Autodesk Inventor part; units mm, degrees
ref_plane "YZ Plane" through (0, 0, 0) normal (1, 0, 0) x (0, 1, 0)
ref_plane "XZ Plane" through (0, 0, 0) normal (0, 1, 0) x (-1, 0, 0)
ref_plane "XY Plane" through (0, 0, 0) normal (0, 0, 1) x (1, 0, 0)
sketch "Sketch1" plane through (0, 0, 0) normal (0, 1, 0) x (-1, 0, 0)
  circle A0 centre (0, 0) radius 6.35
  line L0 (22, 0) -> (6.76, 15.24)
  line L1 (6.76, 15.24) -> (-15.24, 9.525)
  line L2 (-15.24, 9.525) -> (-15.24, 0)
  line L3 (22, 0) -> (0, 0)
  line L4 (22, 0) -> (6.76, -15.24)
  line L5 (6.76, -15.24) -> (-15.24, -9.525)
  line L6 (-15.24, -9.525) -> (-15.24, 0)
  dimension "d0" = 12.7
  dimension "d1" = 22
  dimension "d2" = 15.24
  dimension "d3" = 45
  dimension "d4" = 15.24
  dimension "d5" = 9.525
extrude "Extrusion1" add sketch "Sketch1" along normal blind 6.35
fillet "Fillet1" radius 1.27 5 edges at (-22, 3.175, 0) (-6.76, 3.175, 15.24) (-6.76, 3.175, -15.24) (15.24, 3.175, 9.525) (15.24, 3.175, -9.525)
properties part number "ALIGNMENT JIG 2SCREEN"
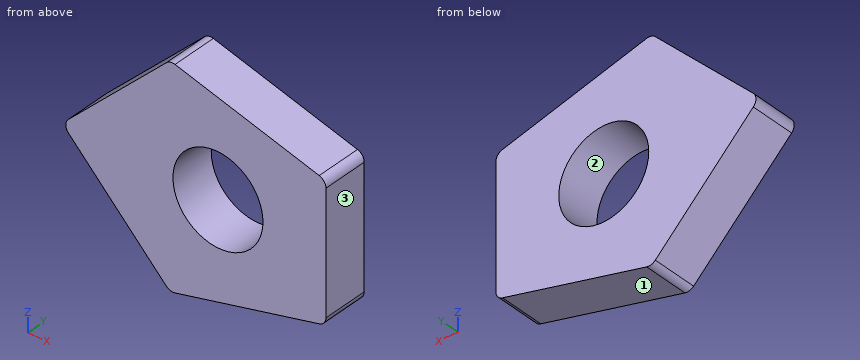
The listing builds one solid part. Answer for the finished solid, in the listing's coordinates (mm). Face numbers are marked on the shaded views. Coordinates: 2 decimals unless noted, no trailing zeros. Order: outer loops, then holes, each group sorted by start corner. A loop starts at its lowest first (then second) coordinate and runs counter-clockwise, first axis right, second up.
Q1. A cutting plane is placed at C-C, the plane x = -0.5. Write down the section's boundary in (y, z), and give its area (3 significant figures).
Q2. Consider line 1 (Z direction, x = -4.5, y = 1); line 2 (Z direction, x = 0, y = 2.25); line 3 (X direction, y = 2, z = -2.5). Determine where each line is inside the solid, lowest interval first.
Q3. A cutting plane is placed at A-A, the plane y = 1. Write down the section's boundary in (x, z), and give its area (3 significant figures).
Q4. Given P1, Ø1, axis at x = 1.5, y = 5, coming from the -Z side; P2, Ø3, axis at x = -8, y = 1, coming from the -Z side, each flat-ended and moving along its own axis, determine where each tip first touches the part or whether it passes through.
Q5. For a pull along Z with two mould halves and no side action, classify the marked faces 1, 2 and 3 as pulls with the +Z half, pulls with the -Z half, needs draft (parallel to the pull), parting line crosses it, or undercut.
Q6. A cutting plane is placed at D-D, the plane x = -11.5. Write down the section's boundary in (y, z), and give its area (3 significant figures).
Q7. A cutting plane is placed at B-B, the plane z = 0. Write down the section's boundary in (x, y).
Answers follow:
1. outline: (0, -13.61) - (6.35, -13.61) - (6.35, -6.33) - (0, -6.33) - close; (0, 6.33) - (6.35, 6.33) - (6.35, 13.61) - (0, 13.61) - close
1. area: 92.5 mm2
2. line 1: z = -14.65 to -4.48, 4.48 to 14.65
2. line 2: z = -13.48 to -6.35, 6.35 to 13.48
2. line 3: x = -19.5 to -5.84, 5.84 to 15.24
3. outline: (-21.1, -0.9) - (-7.27, -14.73) arc R1.27 ccw to (-6.06, -15.06) - (14.29, -9.77) arc R1.27 ccw to (15.24, -8.54) - (15.24, 8.54) arc R1.27 ccw to (14.29, 9.77) - (-6.06, 15.06) arc R1.27 ccw to (-7.27, 14.73) - (-21.1, 0.9) arc R1.27 ccw to start; hole circle Ø12.7 at (0, 0)
3. area: 650 mm2
4. P1: stops at z = -13.22
4. P2: stops at z = -15.09
5. face 1: pulls with the -Z half
5. face 2: undercut
5. face 3: needs draft
6. outline: (0, -10.5) - (6.35, -10.5) - (6.35, 10.5) - (0, 10.5) - close
6. area: 133 mm2
7. outline: (-21.47, 0) - (-6.35, 0) - (-6.35, 6.35) - (-21.47, 6.35) - close; (6.35, 0) - (15.24, 0) - (15.24, 6.35) - (6.35, 6.35) - close
